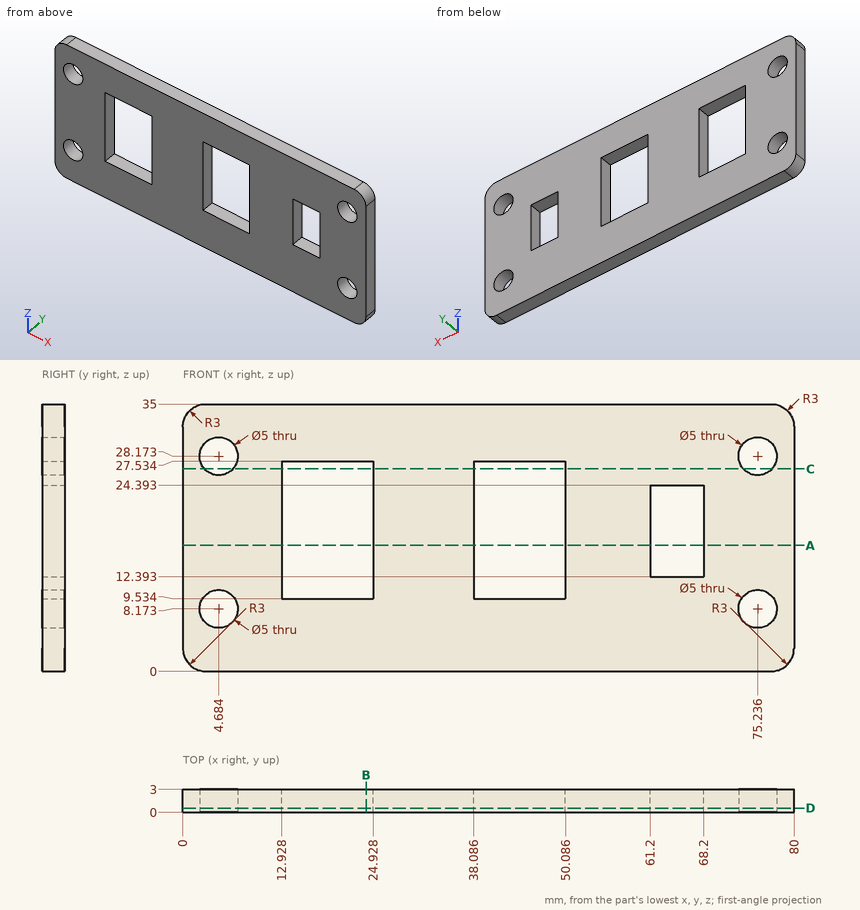
Job drawing, mm, ordinate dimensions from the low corner. One solid piece. Give positions to 0.01 mm unless a question says otherwise; leave off trailing zeros. Loops run counter-clockwise (first coordinate to the right, second up) from the corner with the lowest first, then second, coordinate; pieces in that order, holes last. Notation, with made-up numbers: (44.5, 56) -> (84.5, 56) arc R36 cw to (84.5, 94) -> close; hole circle Ø7 at (71.25, 41.5). An arc over 180 degrees is marked (long way). Write each question's results on one line, items separated by ' | '. Start each with the question number.
Q1. Band-saw the part on D-D on y = 0.55. List the corners of the cut face in (x, z).
Q2. Band-saw the part on C-C on z = 26.5. List the corners of the cut face in (x, y) (1 decimal), plus the area to 3 significant figures.
Q3. Band-saw the part on A-A on z = 16.5. List the corners of the cut face in (x, y).
Q4. Band-saw the part on B-B on x = 24. List the corners of the cut face in (y, z), plus the area to 3 significant figures.
Q5. Wall check: L1, parallel to X at y = 0.95, z = 20; L2, parallel to X at y = 1.2, z = 25; L3, parallel to X at y = 2.7, z = 8. Give the ranges that are in metal, low to high.
Results are:
1) outline: (0, 3) arc R3 ccw to (3, 0) -> (77, 0) arc R3 ccw to (80, 3) -> (80, 32) arc R3 ccw to (77, 35) -> (3, 35) arc R3 ccw to (0, 32) -> close; hole circle Ø5 at (4.68, 8.17); hole circle Ø5 at (4.68, 28.17); hole (12.93, 9.53) -> (24.93, 9.53) -> (24.93, 27.53) -> (12.93, 27.53) -> close; hole (38.09, 9.53) -> (50.09, 9.53) -> (50.09, 27.53) -> (38.09, 27.53) -> close; hole (61.2, 12.39) -> (68.2, 12.39) -> (68.2, 24.39) -> (61.2, 24.39) -> close; hole circle Ø5 at (75.24, 8.17); hole circle Ø5 at (75.24, 28.17)
2) outline: (0, 0) -> (2.8, 0) -> (2.8, 3) -> (0, 3) -> close; (6.5, 0) -> (12.9, 0) -> (12.9, 3) -> (6.5, 3) -> close; (24.9, 0) -> (38.1, 0) -> (38.1, 3) -> (24.9, 3) -> close; (50.1, 0) -> (73.4, 0) -> (73.4, 3) -> (50.1, 3) -> close; (77.1, 0) -> (80, 0) -> (80, 3) -> (77.1, 3) -> close | area: 146 mm²
3) outline: (0, 0) -> (12.93, 0) -> (12.93, 3) -> (0, 3) -> close; (24.93, 0) -> (38.09, 0) -> (38.09, 3) -> (24.93, 3) -> close; (50.09, 0) -> (61.2, 0) -> (61.2, 3) -> (50.09, 3) -> close; (68.2, 0) -> (80, 0) -> (80, 3) -> (68.2, 3) -> close
4) outline: (0, 0) -> (3, 0) -> (3, 9.53) -> (0, 9.53) -> close; (0, 27.53) -> (3, 27.53) -> (3, 35) -> (0, 35) -> close | area: 51.0 mm²
5) L1: x = 0 to 12.93, 24.93 to 38.09, 50.09 to 61.2, 68.2 to 80 | L2: x = 0 to 12.93, 24.93 to 38.09, 50.09 to 80 | L3: x = 0 to 2.19, 7.18 to 72.74, 77.73 to 80
